Work out the finished part from the listing and answer in its coordinate system (mm). Face numbers are marked on the shaded views. A direction names the side the tool comes from. Round coordinates to 2 decimals unless told otherwise and drop trailing zeros. Order: outer loops, then holes, each group sorted by start corner. A loop starts at its lowest first (then second) coordinate and runs counter-clockwise, first axis right, second up. Notation, with made-up numbers: (2, -26.75) - (38, -26.75) arc R25 cw to (38, 12.25) - close; hole circle Ø1 at (19, 57.5). An arc over 180 degrees is marked (long way). One line per question, with ' | ' between items. Start each with the question number.
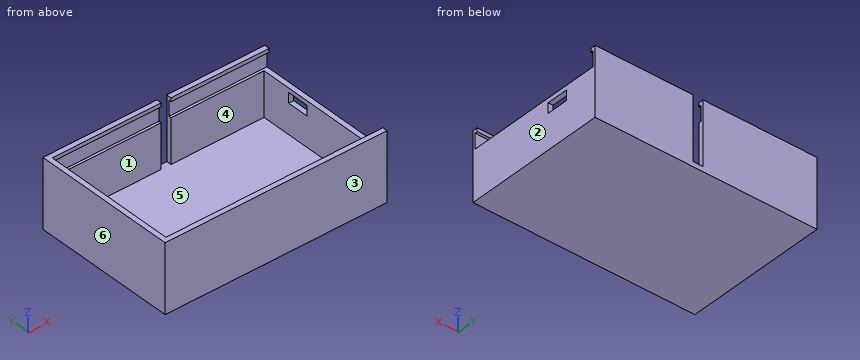
Autodesk Inventor part; units mm, degrees
ref_plane "YZ Plane" through (0, 0, 0) normal (1, 0, 0) x (0, 1, 0)
ref_plane "XZ Plane" through (0, 0, 0) normal (0, 1, 0) x (-1, 0, 0)
ref_plane "XY Plane" through (0, 0, 0) normal (0, 0, 1) x (1, 0, 0)
sketch "Sketch1" plane through (0, 0, 0) normal (0, 0, 1) x (1, 0, 0)
  line L0 (0, 0) -> (83.9978, 0)
  line L1 (83.9978, 0) -> (83.9978, 52.9999)
  line L2 (83.9978, 52.9999) -> (0, 52.9999)
  line L3 (0, 52.9999) -> (0, 0)
  dimension "d0" = 83.9978
  dimension "d1" = 52.9999
extrude "Extrusion1" add sketch "Sketch1" along normal blind 24.9987
shell "Shell1" thickness 1.9812 outward yes removed faces 1 at (55.9985, 17.6666, 24.9987)
sketch "Sketch2" plane through (85.979, -1.9812, -1.9812) normal (1, 0, 0) x (0, 0, -1)
  point P0 (-1.9812, 1.9812)
sketch "Sketch3" plane through (85.979, -1.9812, -1.9812) normal (1, 0, 0) x (0, 0, -1)
  line L0 (-13.7922, 43.5102) -> (-17.78, 43.5102)
  line L1 (-17.78, 43.5102) -> (-17.78, 35.0012)
  line L2 (-17.78, 35.0012) -> (-13.7922, 35.0012)
  line L3 (-13.7922, 35.0012) -> (-13.7922, 43.5102)
  point P0 (-1.9812, 1.9812)
  dimension "d5" = 3.9878
  dimension "d6" = 8.509
extrude "Extrusion2" cut sketch "Sketch3" against normal blind 22.9997
sketch "Sketch4" plane through (85.979, -1.9812, -1.9812) normal (1, 0, 0) x (0, 0, -1)
  line L0 (-19.5072, 55.9816) -> (-25.5072, 55.9816)
  line L1 (-24.5072, 0.9817) -> (-19.5072, 0.9817)
  line L2 (-19.5072, 0.9817) -> (-19.5072, 55.9816)
  line L3 (-25.5072, 55.9816) -> (-19.5072, 55.9816)
  line L4 (-19.5072, 55.9816) -> (-19.5072, 0.9817)
  line L5 (-19.5072, 0.9817) -> (-25.5072, 0.9817)
  line L6 (-25.5072, 0.9817) -> (-25.5072, 55.9816)
  point P0 (-1.9812, 1.9812)
  dimension "d9" = 5
extrude "Extrusion3" cut sketch "Sketch4" against normal blind 87.0001
sketch "Sketch5" plane through (85.979, -0.9995, 17.526) normal (0, 0, 1) x (1, 0, 0)
  point P0 (-85.979, 0.9995)
sketch "Sketch6" plane through (85.979, -1.9812, -1.9812) normal (1, 0, 0) x (0, 0, -1)
  point P0 (-1.9812, 1.9812)
  point P1 (-24.5072, 55.9816)
sketch "Sketch7" plane through (0, 0, 24.9987) normal (0, 0, 1) x (1, 0, 0)
  line L0 (83.9978, 52.9999) -> (0, 52.9999)
  line L1 (85.979, -1.9812) -> (85.979, 54.9811)
  line L2 (83.9978, 52.9999) -> (85.979, 52.9999)
  line L3 (85.979, 52.9999) -> (85.979, 0)
  line L4 (85.979, 0) -> (83.9978, 0)
  line L5 (83.9978, 0) -> (83.9978, 52.9999)
  point P0 (0, 0)
extrude "Extrusion4" cut sketch "Sketch7" against normal blind 2.0066
sketch "Sketch8" plane through (-1.9812, 54.9811, -1.9812) normal (0, 1, 0) x (1, 0, 0)
  line L0 (1.9812, -26.9799) -> (87.9602, -26.9799)
  line L1 (85.979, -1.9812) -> (1.9812, -1.9812)
  line L2 (49.0812, -26.9799) -> (45.1611, -26.9799)
  line L3 (45.1611, -26.9799) -> (45.1611, -1.9812)
  line L4 (45.1611, -1.9812) -> (49.0812, -1.9812)
  line L5 (49.0812, -1.9812) -> (49.0812, -26.9799)
extrude "Extrusion5" cut sketch "Sketch8" against normal blind 25.4
sketch "Sketch9" plane through (85.979, -1.9812, -1.9812) normal (1, 0, 0) x (0, 0, -1)
  point P0 (-1.9812, 1.9812)
properties part number "finalCase"
1) For the marked faces 1 and 2, determine the directions among +Z, -Z, +X, -X, +Y, -Y from which every point of the face is accessible in a straight line to the end or side of a thin tool.
2) Determine the mould class of the marked faces 3, 4, 5 and 6 for opening direction Y: released by +Y, released by -Y, zero draft, split by the parting line, or undercut.
3) Section A-A on z = 20.25 is taken. Give the vertices of the cut face in (x, y).
4) Section B-B on y = 39.5 is taken. Give the vertices of the cut face in (x, z).
5) Section D-D on z = 1.75 is taken. Give the vertices of the cut face in (x, y), and give its area (3 significant figures).
6) Section C-C on y = 23.5 is taken. Give the vertices of the cut face in (x, z).
7) Straight lines are drawn through the part: line 1 (Y direction, x = 71, z = 17); line 2 (X direction, y = 30.5, z = 8.25); line 3 (Y direction, x = 20, z = 18). For each, find the intervals that lie inside material, in ascending order.
8) Flat-ended cylindrical pins translate along their axes: pin 1 (1.6 mm diameter, centred on y = 28, z = 24, fed in from +X); pin 2 (4 mm diameter, centred on x = 37, y = 10, fed in from +Z). Find the tip coordinate at first contact, or state that the pin passes through.
Recorded:
1) face 1: +Z | face 2: +Z, -Z, +X, +Y, -Y
2) face 3: released by -Y | face 4: undercut | face 5: undercut | face 6: zero draft
3) outline: (-1.98, -1.98) - (85.98, -1.98) - (85.98, -1) - (-1.02, -1) - (-1.02, 54) - (43.18, 54) - (43.18, 54.98) - (-1.98, 54.98) - close; (47.1, 54) - (85.98, 54) - (85.98, 54.98) - (47.1, 54.98) - close
4) outline: (-1.98, -1.98) - (85.98, -1.98) - (85.98, 11.81) - (84, 11.81) - (84, 0) - (0, 0) - (0, 17.53) - (-1.02, 17.53) - (-1.02, 23.53) - (0, 23.53) - (0, 25) - (-1.98, 25) - close; (84, 15.8) - (85.98, 15.8) - (85.98, 17.53) - (84, 17.53) - close
5) outline: (-1.98, -1.98) - (85.98, -1.98) - (85.98, 54.98) - (47.1, 54.98) - (47.1, 53) - (84, 53) - (84, 0) - (0, 0) - (0, 53) - (43.18, 53) - (43.18, 54.98) - (-1.98, 54.98) - close | area: 551 mm²
6) outline: (-1.98, -1.98) - (85.98, -1.98) - (85.98, 17.53) - (84, 17.53) - (84, 0) - (0, 0) - (0, 17.53) - (-1.02, 17.53) - (-1.02, 23.53) - (0, 23.53) - (0, 25) - (-1.98, 25) - close
7) line 1: y = -1.98 to 0, 53 to 54.98 | line 2: x = -1.98 to 0, 84 to 85.98 | line 3: y = -1.98 to -1, 54 to 54.98
8) pin 1: stops at x = 0 | pin 2: stops at z = 0
